Answer from the drawing. Dimensions are ordinates in mm from the lowest x, y and z of the part. A direction names the side the tool comes from. Give positions to 0.01 mm unless a question says otherwise; leave off trailing zeros. Order: outer loops, then holes, each group sorted by start corner. A loop starts at its lowest first (then second) coordinate and runs counter-clockwise, first axis right, second up.
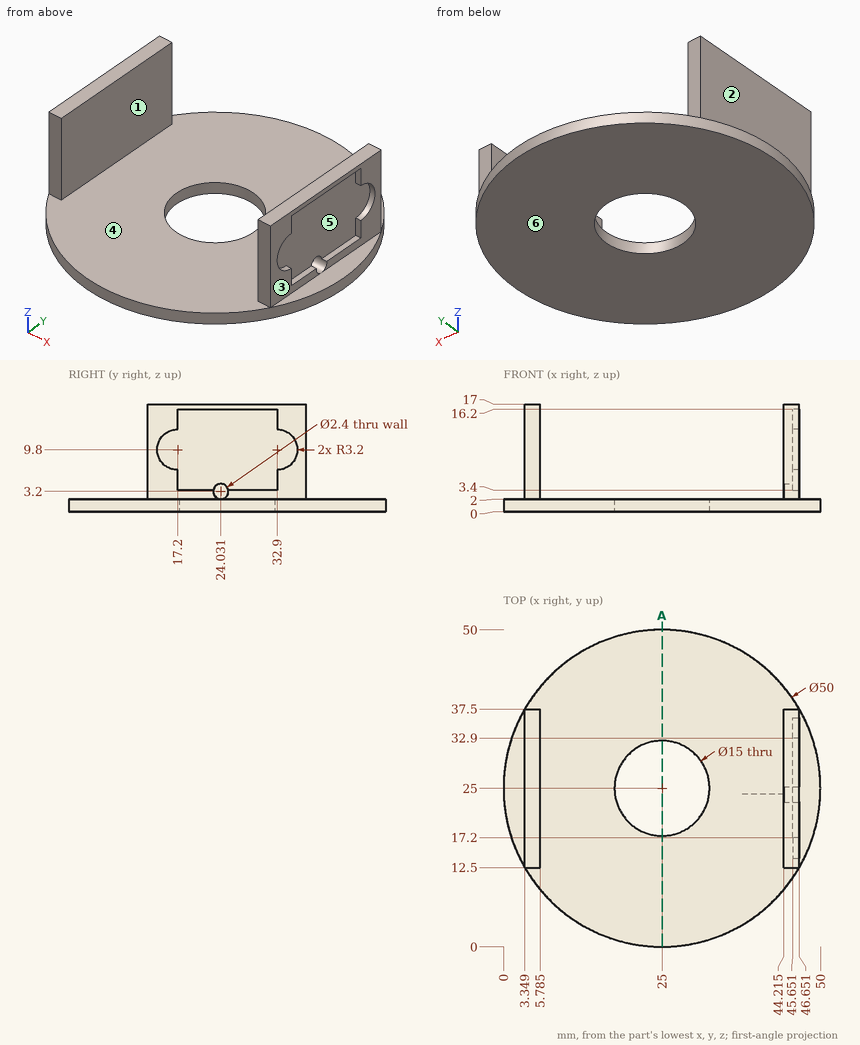
1) Consider L1, parallel to Y at x = 45.55, z = 3.2; L2, parallel to Y at x = 25, z = 1.4; L3, parallel to Z at x = 35.5, y = 14.5. Determine where each line is inside the solid, lowest interval first.
Final values:
L1: y = 12.5 to 22.83, 25.23 to 37.5
L2: y = 0 to 17.5, 32.5 to 50
L3: z = 0 to 2
2) For a pull along X with two mould halves and no side action, classify the marked faces 4, 5 and 6 as released by +X, released by -X, zero draft, split by the parting line, or undercut.
Final values:
face 4: undercut
face 5: released by +X
face 6: zero draft
3) Given pin 1 (0.5 mm diameter, centred on x = 46.5, z = 5.5, fed in from -Y); pin 2 (1.4 mm diameter, centred on y = 24.03, z = 3.2, fed in from +X) (1 decimal); pin 3 (1 mm diameter, centred on x = 17.5, y = 14.5, fed in from +Z); pin 4 (8 mm diameter, centred on y = 5.5, z = 14.5, fed in from -X), each flat-ended and moving along its own axis, determine where each tip first touches the part or whether it passes through.
Final values:
pin 1: stops at y = 12.5
pin 2: stops at x = 5.8
pin 3: stops at z = 2
pin 4: passes through
4) The part is cut by section A-A on x = 25. Determine the outline of the cut face in (y, z).
Final values:
outline: (0, 0) - (17.5, 0) - (17.5, 2) - (0, 2) - close; (32.5, 0) - (50, 0) - (50, 2) - (32.5, 2) - close
5) A tool of negligible diameter and unlimited length cuts with its end or side. For the marked faces 1, 2 and 3, from which of +Z, -Z, +X, -X, +Y, -Y can it reach the whole face along a straight path? Write none if from no direction.
Final values:
face 1: +Z, +Y, -Y
face 2: +Z, -X, +Y, -Y
face 3: +Z, +X, +Y, -Y
